```python
from build123d import *

# Parameters (mm, degrees)
SKETCH1_W           = 47
SKETCH1_H           = 58
BOSS_EXTRUDE1_DEPTH = 16
FILLET1_R           = 8
SKETCH2_W           = 14
SKETCH2_H           = 52
CUT_EXTRUDE1_DEPTH  = 14
CUT_EXTRUDE2_REACH  = 47.708
SKETCH4_R           = 7.25
BOSS_EXTRUDE3_DEPTH = 24
SKETCH5_R           = 2.4
SKETCH5_R_2         = 1.2
BOSS_EXTRUDE4_DEPTH = 1.5
SKETCH6_R           = 1
BOSS_EXTRUDE5_DEPTH = 2.5


with BuildPart() as part:
    # Sketch1 → Boss-Extrude1 (new body)
    with BuildSketch(Plane(origin=(0, 0, 0), x_dir=(1, 0, 0), z_dir=(0, 1, 0))):
        Rectangle(SKETCH1_W, SKETCH1_H)
    extrude(amount=BOSS_EXTRUDE1_DEPTH)

    # Fillet1
    fillet1_edges = [part.edges().sort_by_distance(p)[0] for p in [
        (-23.5, 16, 0),
        (23.5, 16, 0),
    ]]
    fillet(fillet1_edges, radius=FILLET1_R)

    # Sketch2 → Cut-Extrude1 (cut)
    with BuildSketch(Plane(origin=(0, 16, 0), x_dir=(1, 0, 0), z_dir=(0, 1, 0))):
        Polygon((-22, 26), (-8, 26), (-8, -26), (-22, -26), (-22, -23.5), (-18.4, -23.5), (-18.4, -8.5), (-22, -8.5), (-22, 8.5), (-18.4, 8.5), (-18.4, 23.5), (-22, 23.5), align=None)
        Rectangle(SKETCH2_W, SKETCH2_H)
        Polygon((8, 26), (22, 26), (22, 23.5), (18.4, 23.5), (18.4, 8.5), (22, 8.5), (22, -8.5), (18.4, -8.5), (18.4, -23.5), (22, -23.5), (22, -26), (8, -26), align=None)
    extrude(amount=-CUT_EXTRUDE1_DEPTH, mode=Mode.SUBTRACT)

    # Cut-Extrude2: up to this face of the body (flat: up to its plane)
    cut_extrude2_end = Plane(part.part.faces().sort_by_distance((-8, 9, 0))[0])
    # Sketch3 → Cut-Extrude2 (cut, up to the picked face)
    with BuildSketch(Plane(origin=(8, 0, 0), x_dir=(0, 0, -1), z_dir=(1, 0, 0)), mode=Mode.PRIVATE) as cut_extrude2_sk1:
        Polygon((-26, 16), (-26, 13.5), (-17.5, 8.2), (17.5, 8.2), (26, 13.5), (26, 16), align=None)
    cut_extrude2_tool1 = split(extrude(cut_extrude2_sk1.sketch, amount=-CUT_EXTRUDE2_REACH, mode=Mode.PRIVATE), bisect_by=cut_extrude2_end, keep=Keep.BOTH, mode=Mode.PRIVATE)
    add(cut_extrude2_tool1.solids().sort_by(Axis((8, 12.366556, 0), (-1, 0, 0)))[0], mode=Mode.SUBTRACT)

    # Sketch4 → Boss-Extrude3 (add, symmetric)
    with BuildSketch(Plane.XY):
        with Locations((-15, 8.75)):
            Circle(SKETCH4_R)
        with Locations((0, 8.75)):
            Circle(SKETCH4_R)
        with Locations((15, 8.75)):
            Circle(SKETCH4_R)
    extrude(amount=BOSS_EXTRUDE3_DEPTH, both=True)

    # Sketch5 → Boss-Extrude4 (add)
    # profile 1 of 3: a face of its own
    with BuildSketch(Plane.XZ):
        with Locations(Location((-19.6, 0, 0), (0, 0, 270))):
            Circle(SKETCH5_R)
        with Locations(Location((-19.6, 0, 0), (0, 0, 270))):
            Circle(SKETCH5_R_2, mode=Mode.SUBTRACT)
    # profile 2 of 3: a face of its own
    with BuildSketch(Plane.XZ):
        with Locations(Location((19.6, 0, 0), (0, 0, 90))):
            Circle(SKETCH5_R)
        with Locations(Location((19.6, 0, 0), (0, 0, 90))):
            Circle(SKETCH5_R_2, mode=Mode.SUBTRACT)
    # profile 3 of 3: a face of its own
    with BuildSketch(Plane.XZ):
        Polygon((-18.8, -26), (12.386677769, 26), (18.8, 26), (-12.386677769, -26), align=None)
    extrude(amount=BOSS_EXTRUDE4_DEPTH)

    # Sketch6 → Boss-Extrude5 (add)
    with BuildSketch(Plane.XY.offset(29)):
        with Locations(Location((-15.5, 2.5, 0), (0, 0, 180))):
            Circle(SKETCH6_R)
        with Locations(Location((-6.8, 2.5, 0), (0, 0, 180))):
            Circle(SKETCH6_R)
    extrude(amount=BOSS_EXTRUDE5_DEPTH)


solid = part.part
```
Read the model definition and answer for the solid it produces. Units are mm, in the model's axes. A direction names the side the tool comes from. Give positions to 0.01 mm unless a question says otherwise; leave off trailing zeros. Order: outer loops, then holes, each group sorted by start corner. A loop starts at its lowest first (then second) coordinate and runs counter-clockwise, first axis right, second up.
(1) Find section B-B (z = 9.5). Give the number of separate pieces and of enclosed holes in the cut face, plus the area to 3 significant figures.
(2) Given pin 1 (5 mm diameter, centred on x = 12, z = 6.5, fed in from +Y); pin 2 (10 mm diameter, centred on x = 2.5, y = 11.5, fed in from +Z); pin 3 (1.6 mm diameter, centred on x = -14.5, y = -0.5, fed in from -Z); pin 4 (1.6 mm diameter, centred on y = 12, z = 3.5, fed in from +X), each flat-ended and moving along its own axis, determine where each tip first touches the part or whether it passes through.
(3) For faces 1 (the flat face through (20, 0, 0)), 2 (the flat face through (0, 9, 26)), 3 (the cylindrical face through (19.84, 3.35, 0.34)), determine the directions among +Z, -Z, +X, -X, +Y, -Y from which every point of the face is accessible in a straight line to the end or side of a thin tool.
(4) Find section A-A (x = 9.5). Give the vertices of the cut face in (y, z), plus the area to 3 significant figures.
(5) Find section C-C (x = 1.5). Give the vertices of the cut face in (y, z).
(6) For a pull along X with two mould halves and no side action, classify faces 4 (the cylindrical face through (22.787, 11.301, -0.406)), 5 (the flat face through (0, 16, 27)), 6 (the flat face through (22, 7, 25)) as released by +X, released by -X, zero draft, split by the parting line, or undercut.
(7) Straight lines are drawn through the part: L1, parallel to X at y = 2.25, z = -25; L2, parallel to Z at x = -10.5, y = 8.75; L3, parallel to X at y = -0.25, z = 0. For each, find the intervals that lie inside material, in ascending order.
Result sheet:
1. separate pieces: 1
1. enclosed holes: 6
1. area: 651 mm2
2. pin 1: stops at y = 15.98
2. pin 2: stops at z = 29
2. pin 3: stops at z = -29
2. pin 4: stops at x = 22.83
3. face 1: -Y
3. face 2: +Y
3. face 3: none
4. outline: (-1.5, 10.49) - (0, 10.49) - (0, -29) - (16, -29) - (16, -26) - (2, -26) - (2, 26) - (16, 26) - (16, 29) - (0, 29) - (0, 21.19) - (-1.5, 21.19) - close; (4.03, -24) - (13.47, -24) - (13.47, 24) - (4.03, 24) - close
4. area: 670 mm2
5. outline: (-1.5, -2.85) - (0, -2.85) - (0, -29) - (16, -29) - (16, -26) - (2, -26) - (2, -24) - (15.84, -24) - (15.84, 24) - (2, 24) - (2, 26) - (16, 26) - (16, 29) - (0, 29) - (0, 7.85) - (-1.5, 7.85) - close
6. face 4: released by +X
6. face 5: zero draft
6. face 6: undercut
7. L1: x = -23.5 to -22, -8 to -7, 7 to 8, 22 to 23.5
7. L2: z = -29 to -26, -24 to 24, 26 to 29
7. L3: x = -22 to -20.8, -18.4 to -17.2, -3.21 to 3.21, 17.2 to 18.4, 20.8 to 22
